Geometry: see drawing. Coordinates: mm, zero at the bounding-box minimum. A direction names the side the tool comes from. Give positions to 0.01 mm unless a question says otherwise; leave off trailing zeros. Order: outer loops, then holes, each group sorted by start corner. A loop starts at its lowest first (then second) coordinate and runs counter-clockwise, first axis right, second up. Notation, with made-up numbers: M 24.25,29 L 56.25,29 A8 ccw 56.25,44 Z; hole C 54.5,-32 d11. An arc over 180 degrees is marked long. Return JSON: item names as keys, results as strings.
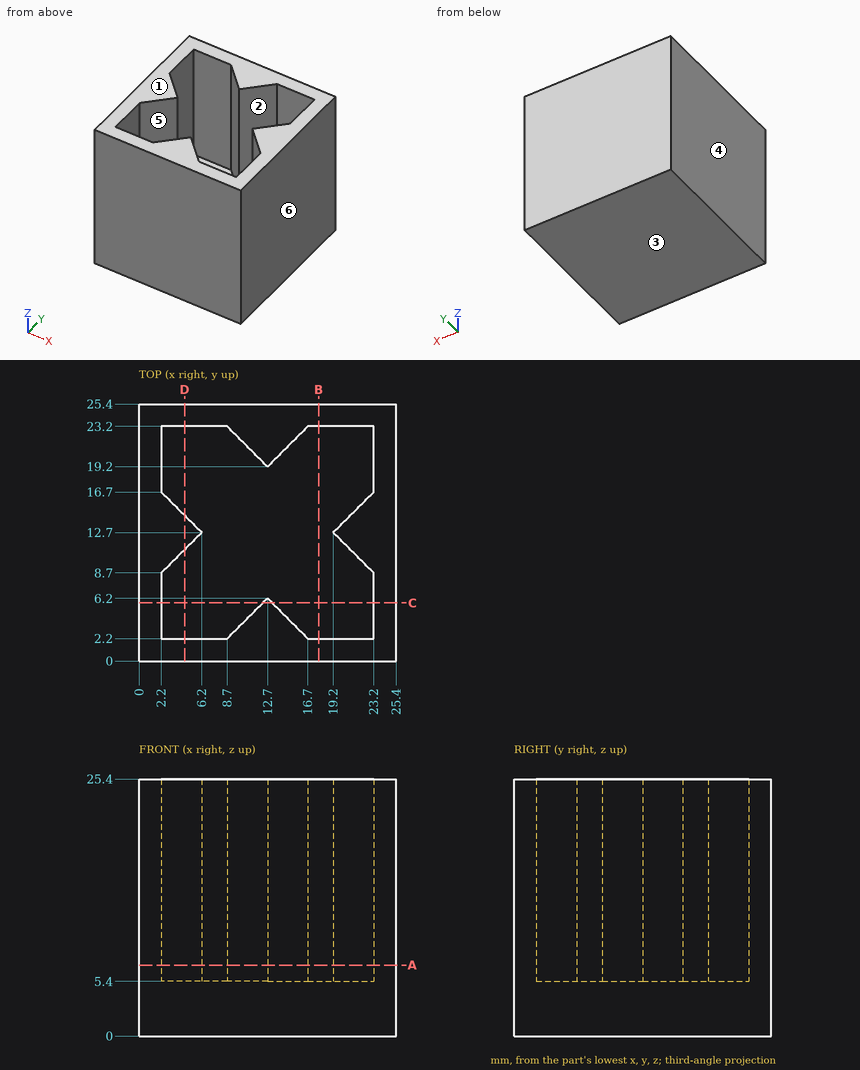
1. Set-up query: the marked faces 1 and 2. Return all of +Z, -Z, +X, -X, +Y, -Y with unobstructed straight access to the full face (end or side cutting, diameter ignored); none if empty.
Evaluation:
{"face 1": "+Z, +X, -X, +Y, -Y", "face 2": "+Z"}
2. Section query D-D (x = 4.5). Return loops of the section in (y, z), then the cut area to 3 significant figures.
Evaluation:
{"outline": "M 0,0 L 25.4,0 L 25.4,25.4 L 23.2,25.4 L 23.2,5.4 L 14.4,5.4 L 14.4,25.4 L 11,25.4 L 11,5.4 L 2.2,5.4 L 2.2,25.4 L 0,25.4 Z", "area": "293 mm^2"}
3. Section query A-A (z = 7). Return loops of the section in (x, y), then the cut area to 3 significant figures.
Evaluation:
{"outline": "M 0,0 L 25.4,0 L 25.4,25.4 L 0,25.4 Z; hole M 2.2,2.2 L 8.7,2.2 L 12.7,6.2 L 16.7,2.2 L 23.2,2.2 L 23.2,8.7 L 19.2,12.7 L 23.2,16.7 L 23.2,23.2 L 16.7,23.2 L 12.7,19.2 L 8.7,23.2 L 2.2,23.2 L 2.2,16.7 L 6.2,12.7 L 2.2,8.7 Z", "area": "268 mm^2"}
4. First-contact query: pin 1 (6.5 mm diameter, centred on x = 14.5, y = 10, fed in from +Z). Flat tip, straight axial feed; report the tip coordinate or a pass-through.
Evaluation:
{"pin 1": "stops at z = 5.4"}
5. Ray query, probe 1 along X at (y, z) = (18.5, 11); probe 2 along Y at (x, z) = (2.5, 9); probe 3 along X at (y, z) = (5, 11.25). Return the intervals inside material, ascending.
Evaluation:
{"probe 1": "x = 0 to 2.2, 23.2 to 25.4", "probe 2": "y = 0 to 2.2, 9 to 16.4, 23.2 to 25.4", "probe 3": "x = 0 to 2.2, 11.5 to 13.9, 23.2 to 25.4"}
6. Section query C-C (y = 5.75). Return loops of the section in (x, z), then the cut area to 3 significant figures.
Evaluation:
{"outline": "M 0,0 L 25.4,0 L 25.4,25.4 L 23.2,25.4 L 23.2,5.4 L 13.15,5.4 L 13.15,25.4 L 12.25,25.4 L 12.25,5.4 L 2.2,5.4 L 2.2,25.4 L 0,25.4 Z", "area": "243 mm^2"}
7. Draft query along X for the marked faces 3, 4, 5 and 6. Return one class per face: pulls with the +X half, pulls with the -X half, needs draft (parallel to the pull), parting line crosses it, or undercut.
Evaluation:
{"face 3": "needs draft", "face 4": "pulls with the -X half", "face 5": "undercut", "face 6": "pulls with the +X half"}
8. Section query B-B (x = 17.75). Return loops of the section in (y, z), then the cut area to 3 significant figures.
Evaluation:
{"outline": "M 0,0 L 25.4,0 L 25.4,25.4 L 23.2,25.4 L 23.2,5.4 L 2.2,5.4 L 2.2,25.4 L 0,25.4 Z", "area": "225 mm^2"}
